```python
from build123d import *

# Parameters (mm, degrees)
SKETCH1_W           = 15
SKETCH1_H           = 10
BOSS_EXTRUDE1_DEPTH = 10
SKETCH2_W           = 0.4
SKETCH2_H           = 8
SKETCH2_W_2         = 0.3
SKETCH2_W_3         = 0.25
CUT_EXTRUDE1_DEPTH  = 5
BOSS_EXTRUDE2_DEPTH = 5
CUT_EXTRUDE2_DEPTH  = 5


with BuildPart() as part:
    # Sketch1 → Boss-Extrude1 (new body)
    with BuildSketch(Plane(origin=(0, 0, 0), x_dir=(1, 0, 0), z_dir=(0, 1, 0))):
        Rectangle(SKETCH1_W, SKETCH1_H)
    extrude(amount=BOSS_EXTRUDE1_DEPTH)

    # Sketch2 → Cut-Extrude1 (cut)
    with BuildSketch(Plane(origin=(0, 10, 0), x_dir=(1, 0, 0), z_dir=(0, 1, 0))):
        with Locations((-4.8, 1)):
            Rectangle(SKETCH2_W, SKETCH2_H)
        with Locations((-1.45, 1)):
            Rectangle(SKETCH2_W_2, SKETCH2_H)
        with Locations((2.1, 1)):
            Rectangle(SKETCH2_W_2, SKETCH2_H)
        with Locations((4.875, 1)):
            Rectangle(SKETCH2_W_3, SKETCH2_H)
    extrude(amount=-CUT_EXTRUDE1_DEPTH, mode=Mode.SUBTRACT)

    # Sketch3 → Boss-Extrude2 (add)
    with BuildSketch(Plane(origin=(0, 10, 0), x_dir=(1, 0, 0), z_dir=(0, 1, 0))):
        with BuildLine():
            Line((-5, 3.4), (-5, 2.25))
            ThreePointArc((-5, 2.25), (-4.90568901, 2.825), (-5, 3.4))
        make_face()
        with BuildLine():
            Line((-5, 0.25), (-5, -0.9))
            ThreePointArc((-5, -0.9), (-4.90568901, -0.325), (-5, 0.25))
        make_face()
        with BuildLine():
            Line((-1.6, 3.4), (-1.6, 2.25))
            ThreePointArc((-1.6, 2.25), (-1.50568901, 2.825), (-1.6, 3.4))
        make_face()
        with BuildLine():
            Line((-1.6, 0.25), (-1.6, -0.9))
            ThreePointArc((-1.6, -0.9), (-1.50568901, -0.325), (-1.6, 0.25))
        make_face()
    extrude(amount=-BOSS_EXTRUDE2_DEPTH)

    # Sketch4 → Cut-Extrude2 (cut)
    with BuildSketch(Plane(origin=(0, 10, 0), x_dir=(1, 0, 0), z_dir=(0, 1, 0))):
        with BuildLine():
            Line((-4.6, 3.4), (-4.6, 2.25))
            ThreePointArc((-4.6, 2.25), (-4.50568901, 2.825), (-4.6, 3.4))
        make_face()
        with BuildLine():
            Line((-4.6, 0.25), (-4.6, -0.9))
            ThreePointArc((-4.6, -0.9), (-4.50568901, -0.325), (-4.6, 0.25))
        make_face()
        with BuildLine():
            Line((-1.3, 3.4), (-1.3, 2.25))
            ThreePointArc((-1.3, 2.25), (-1.20568901, 2.825), (-1.3, 3.4))
        make_face()
        with BuildLine():
            Line((-1.3, 0.25), (-1.3, -0.9))
            ThreePointArc((-1.3, -0.9), (-1.20568901, -0.325), (-1.3, 0.25))
        make_face()
    extrude(amount=-CUT_EXTRUDE2_DEPTH, mode=Mode.SUBTRACT)


solid = part.part
```
The listing builds one solid part. Answer for the finished solid, in the listing's coordinates (mm). A direction names the side the tool comes from. Coordinates: 2 decimals unless noted, no trailing zeros. Write each loop counter-clockwise with the first axis right and the second up, starting at its lowest first coordinate (ties: lowest second). Pieces come first, ordered by that corner, then holes. Notation, with made-up numbers: (-24.75, 28.25) - (-4.75, 28.25) arc R20 ccw to (-4.75, 47.25) - close; hole circle Ø6 at (22.5, -10.5). An arc over 180 degrees is marked (long way). One line per item, written item: value.
1) Find section A-A (z = -2). Give the vertices of the cut face in (x, y).
Geometry check:
outline: (-7.5, 0) - (7.5, 0) - (7.5, 10) - (5, 10) - (5, 5) - (4.75, 5) - (4.75, 10) - (2.25, 10) - (2.25, 5) - (1.95, 5) - (1.95, 10) - (-1.3, 10) - (-1.3, 5) - (-1.6, 5) - (-1.6, 10) - (-4.6, 10) - (-4.6, 5) - (-5, 5) - (-5, 10) - (-7.5, 10) - close
2) A tool of negligible diameter and unlimited length cuts with its end or side. For faces 5 (the flat face through (7.5, 5, 0)), 6 (the flat face through (2.25, 8, -1)), 7 (the flat face through (-5, 8, -1)), from which of +Z, -Z, +X, -X, +Y, -Y can it reach the whole face along a straight path? Write none if from no direction.
Geometry check:
face 5: +Z, -Z, +X, +Y, -Y
face 6: -Z, +Y
face 7: +Y
3) Consider line 1 along X through (y, z) = (5.75, -1.5); line 2 along X through (y, z) = (5.5, 0.5); line 3 along Y through (x, z) = (-1.5, 1.75). Determine where each line is inside the solid, lowest interval first. Write a range as from..to.
Geometry check:
line 1: x = -7.5..-5, -4.6..-1.6, -1.3..1.95, 2.25..4.75, 5..7.5
line 2: x = -7.5..-4.91, -4.51..-1.51, -1.21..1.95, 2.25..4.75, 5..7.5
line 3: y = 0..5
4) For a pull along Z with two mould halves and no side action, classify faces 1 (the flat face through (0, 5, 5)), 2 (the cylindrical face through (-1.506, 7.535, 0.333)), 3 (the cylindrical face through (-1.206, 7.535, -2.817)), 4 (the flat face through (-1.3, 8, 2)) as pulls with the +Z half, pulls with the -Z half, needs draft (parallel to the pull), parting line crosses it, or undercut.
Geometry check:
face 1: pulls with the +Z half
face 2: undercut
face 3: undercut
face 4: needs draft
